Geometry: see drawing. Coordinates: mm, zero at the bounding-box minimum. Give positions to 0.01 mm unless a question says otherwise; leave off trailing zeros. Write each loop counter-clockwise with the first axis right and the second up, starting at its lowest first coordinate (ties: lowest second). Pieces come first, ordered by that corner, then holes. Notation, with made-up numbers: (35, -36.5) - (80, -36.5) arc R30 cw to (80, -0.5) - close; hole circle Ø7 at (60.25, 50.5). An arc over 180 degrees is marked (long way). Use a Markdown table: item, result. Add a question column.
1. Section query C-C, the plane x = 67. Return loops of the section in (y, z).
2. Pin query (flat end, axial travel): pin 1 (5 mm diameter, centred on x = 38.5, y = 34, fed in from -Z); pin 2 (12 mm diameter, centred on x = 29.5, z = 26.5, fed in from +Y); pin 3 (1.5 mm diameter, centred on y = 75.5, z = 19.5, fed in from +X). Return the tip coordinate at first contact, or that it passes through.
3. Material intervals for probe 1 along X at (y, z) = (25.5, 16.5); probe 2 along Y at (x, z) = (21.5, 31); probe 3 along Y at (x, z) = (78, 4), sorted ascending.
4. Section query A-A, the plane z = 27. Return loops of the section in (x, y) (3 decimals), plus the area to 3 significant figures.
5. Section query B-B, the plane y = 62.5. Return loops of the section in (x, z), plus the area to 3 significant figures.
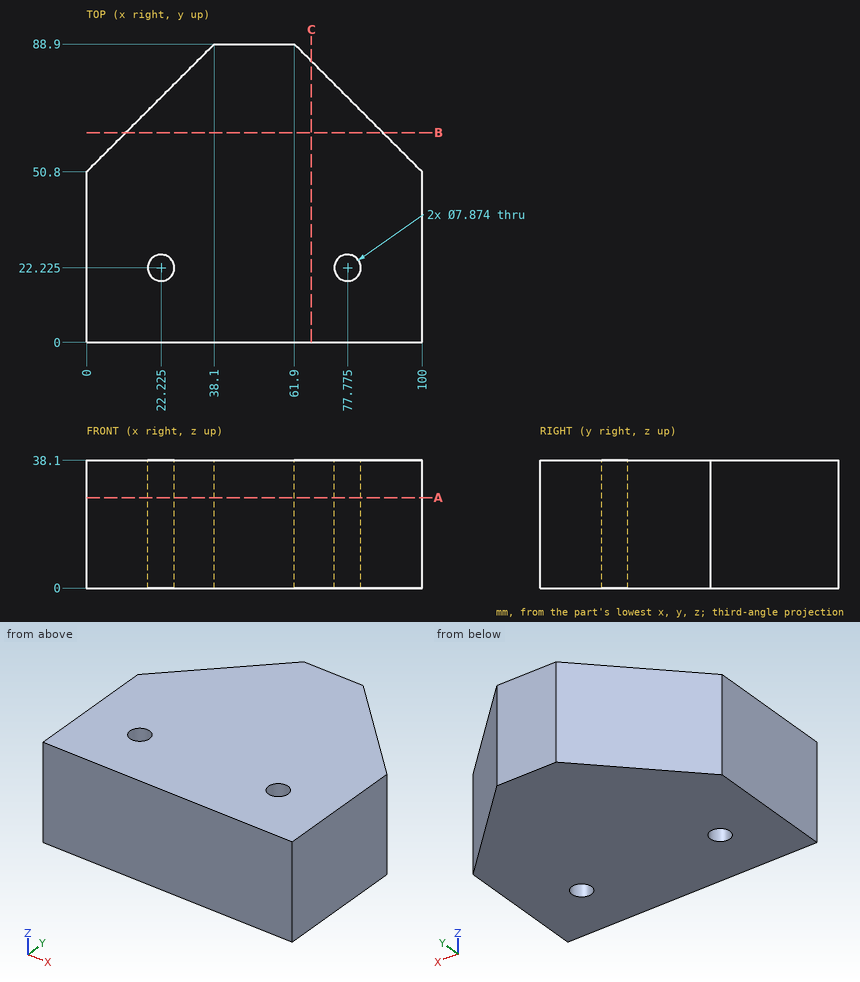
Result sheet:
| question | item | result |
|---|---|---|
| 1 | outline | (0, 0) - (83.8, 0) - (83.8, 38.1) - (0, 38.1) - close |
| 2 | pin 1 | stops at z = 0 |
| 2 | pin 2 | stops at y = 86.3 |
| 2 | pin 3 | stops at x = 76.05 |
| 3 | probe 1 | x = 0 to 20.04, 24.41 to 75.59, 79.96 to 100 |
| 3 | probe 2 | y = 0 to 18.36, 26.09 to 72.3 |
| 3 | probe 3 | y = 0 to 18.29, 26.16 to 72.8 |
| 4 | outline | (0, 0) - (100, 0) - (100, 50.8) - (61.9, 88.9) - (38.1, 88.9) - (0, 50.8) - close; hole circle Ø7.874 at (22.225, 22.225); hole circle Ø7.874 at (77.775, 22.225) |
| 4 | area | 7,340 mm² |
| 5 | outline | (11.7, 0) - (88.3, 0) - (88.3, 38.1) - (11.7, 38.1) - close |
| 5 | area | 2,920 mm² |
